Autodesk Inventor part; units mm, degrees
ref_plane "YZ Plane" through (0, 0, 0) normal (1, 0, 0) x (0, 1, 0)
ref_plane "XZ Plane" through (0, 0, 0) normal (0, 1, 0) x (-1, 0, 0)
ref_plane "XY Plane" through (0, 0, 0) normal (0, 0, 1) x (1, 0, 0)
sketch "Sketch1" plane through (0, 0, 0) normal (0, 0, 1) x (1, 0, 0)
  line L0 (-314, 325.9188) -> (-204, 325.9188)
  line L1 (-204, 325.9188) -> (-204, 545.9188)
  line L2 (-204, 545.9188) -> (-424, 545.9188)
  line L3 (-424, 545.9188) -> (-424, 325.9188)
  line L4 (-424, 325.9188) -> (-314, 325.9188)
  line L5 (0, 0) -> (100, 30)
  line L6 (0, 0) -> (272.914, 0) construction
  line L7 (100, 30) -> (100, 605)
  line L8 (0, 0) -> (-550, 0)
  line L9 (-550, 0) -> (-550, 605)
  line L10 (100, 605) -> (-90.9188, 795.9188)
  line L11 (100, 605) -> (370, 605) construction
  line L12 (-90.9188, 795.9188) -> (-359.0812, 795.9188)
  line L13 (-550, 605) -> (-359.0812, 795.9188)
  line L14 (-550, 605) -> (-280, 605) construction
  dimension "d10" = 110
  dimension "d11" = 220
  dimension "d12" = 220
  dimension "d21" = 100
  dimension "d24" = 550
  dimension "d25" = 126
  dimension "d29" = 30
  dimension "d30" = 270
  dimension "d31" = 135
  dimension "d32" = 270
  dimension "d33" = 45
  dimension "d34" = 605
  dimension "d35" = 250
extrude "Extrusion1" add sketch "Sketch1" along normal blind 1.6
fillet "Fillet2" radius 30 2 edges at (100, 605, 0.8) (-90.9188, 795.9188, 0.8)
equation "\"BendRadius\" = Thickness"
equation "\"BendReliefWidth\" = Thickness"
equation "\"BendReliefDepth\" = 0.5 * Thickness"
equation "\"CornerReliefSize\" = 4 * Thickness"
equation "\"MinimumRemnant\" = 2 * Thickness"
equation "\"TransitionRadius\" = BendRadius"
equation "\"JacobiRadiusSize\" = Thickness"
equation "\"GapSize\" = Thickness"
properties part number "side plate" material "Steel"
The model under review builds one solid part; all positions refer to its coordinate system, in mm. Round coordinates to 2 decimals unless told otherwise and drop trailing zeros. Order: outer loops, then holes, each group sorted by start corner. A loop starts at its lowest first (then second) coordinate and runs counter-clockwise, first axis right, second up.
Item 1: Add section A-A, the plane y = 529. State the section outline as (x, z) points.
Working result:
outline: (-550, 0) - (-424, 0) - (-424, 1.6) - (-550, 1.6) - close; (-204, 0) - (100, 0) - (100, 1.6) - (-204, 1.6) - close
Item 2: Add section C-C, the plane z = 1.1. State the section outline as (x, y) points, and give its area (3 significant figures).
Working result:
outline: (-550, 0) - (0, 0) - (100, 30) - (100, 592.57) arc R30 ccw to (91.21, 613.79) - (-82.13, 787.13) arc R30 ccw to (-103.35, 795.92) - (-359.08, 795.92) - (-550, 605) - close; hole (-424, 325.92) - (-204, 325.92) - (-204, 545.92) - (-424, 545.92) - close
area: 431,000 mm2
Item 3: To check wall thickness, follow probe 1 along Y at (x, z) = (-228, 0.3); probe 2 along X at (y, z) = (359.5, 0.1); probe 3 along Y at (x, z) = (-383.5, 1.1). State the ranges of each line that lie inside material, in increasing order.
Working result:
probe 1: y = 0 to 325.92, 545.92 to 795.92
probe 2: x = -550 to -424, -204 to 100
probe 3: y = 0 to 325.92, 545.92 to 771.5
Item 4: Add section B-B, the plane x = -405. State the section outline as (y, z) points, and give its area (3 significant figures).
Working result:
outline: (0, 0) - (325.92, 0) - (325.92, 1.6) - (0, 1.6) - close; (545.92, 0) - (750, 0) - (750, 1.6) - (545.92, 1.6) - close
area: 848 mm2
Item 5: Add section D-D, the plane x = -494.5. State the section outline as (y, z) points, and give its area (3 significant figures).
Working result:
outline: (0, 0) - (660.5, 0) - (660.5, 1.6) - (0, 1.6) - close
area: 1,060 mm2
